The listing builds one solid part. Answer for the finished solid, in the listing's coordinates (mm). Give positions to 0.01 mm unless a question says otherwise; leave off trailing zeros. Write each loop counter-clockwise with the first axis right and the second up, starting at its lowest first coordinate (ties: lowest second). Pieces come first, ordered by that corner, then holes.
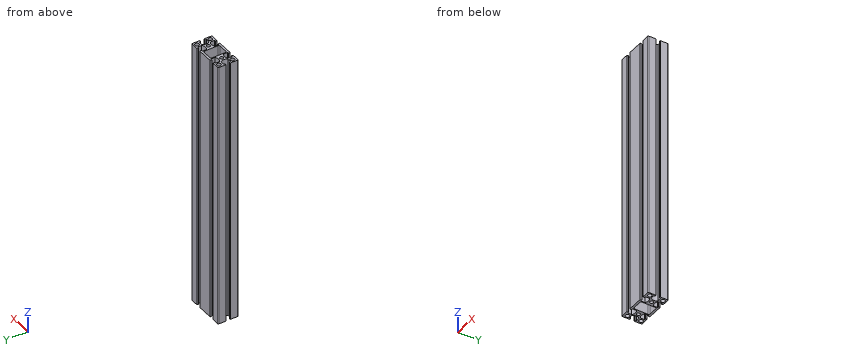
```python
from build123d import *

# Parameters (mm, degrees)
MODEL_R             = 2.5
MODEL_R_2           = 3
BOSS_EXTRUDE1_DEPTH = 400


with BuildPart() as part:
    # Model → Boss-Extrude1 (new body)
    with BuildSketch(Plane.XY):
        with BuildLine():
            Line((-27.5, 3.25), (-30, 3.25))
            Line((-30, 3.25), (-30, 14))
            ThreePointArc((-30, 14), (-29.707106781, 14.707106781), (-29, 15))
            Line((-29, 15), (-18.25, 15))
            Line((-18.25, 15), (-18.25, 12.5))
            Line((-18.25, 12.5), (-20.25, 12.5))
            Line((-20.25, 12.5), (-20.25, 6.643928679))
            ThreePointArc((-20.25, 6.643928679), (-15, 4.5), (-9.75, 6.643928679))
            Line((-9.75, 6.643928679), (-9.75, 12.5))
            Line((-9.75, 12.5), (-11.75, 12.5))
            Line((-11.75, 12.5), (-11.75, 15))
            Line((-11.75, 15), (11.75, 15))
            Line((11.75, 15), (11.75, 12.5))
            Line((11.75, 12.5), (9.75, 12.5))
            Line((9.75, 12.5), (9.75, 6.643928679))
            ThreePointArc((9.75, 6.643928679), (15, 4.5), (20.25, 6.643928679))
            Line((20.25, 6.643928679), (20.25, 12.5))
            Line((20.25, 12.5), (18.25, 12.5))
            Line((18.25, 12.5), (18.25, 15))
            Line((18.25, 15), (29, 15))
            ThreePointArc((29, 15), (29.707106781, 14.707106781), (30, 14))
            Line((30, 14), (30, 3.25))
            Line((30, 3.25), (27.5, 3.25))
            Line((27.5, 3.25), (27.5, 5.25))
            Line((27.5, 5.25), (21.643928679, 5.25))
            ThreePointArc((21.643928679, 5.25), (19.5, 0), (21.643928679, -5.25))
            Line((21.643928679, -5.25), (27.5, -5.25))
            Line((27.5, -5.25), (27.5, -3.25))
            Line((27.5, -3.25), (30, -3.25))
            Line((30, -3.25), (30, -14))
            ThreePointArc((30, -14), (29.707106781, -14.707106781), (29, -15))
            Line((29, -15), (18.25, -15))
            Line((18.25, -15), (18.25, -12.5))
            Line((18.25, -12.5), (20.25, -12.5))
            Line((20.25, -12.5), (20.25, -6.643928679))
            ThreePointArc((20.25, -6.643928679), (15, -4.5), (9.75, -6.643928679))
            Line((9.75, -6.643928679), (9.75, -12.5))
            Line((9.75, -12.5), (11.75, -12.5))
            Line((11.75, -12.5), (11.75, -15))
            Line((11.75, -15), (-11.75, -15))
            Line((-11.75, -15), (-11.75, -12.5))
            Line((-11.75, -12.5), (-9.75, -12.5))
            Line((-9.75, -12.5), (-9.75, -6.643928679))
            ThreePointArc((-9.75, -6.643928679), (-15, -4.5), (-20.25, -6.643928679))
            Line((-20.25, -6.643928679), (-20.25, -12.5))
            Line((-20.25, -12.5), (-18.25, -12.5))
            Line((-18.25, -12.5), (-18.25, -15))
            Line((-18.25, -15), (-29, -15))
            ThreePointArc((-29, -15), (-29.707106781, -14.707106781), (-30, -14))
            Line((-30, -14), (-30, -3.25))
            Line((-30, -3.25), (-27.5, -3.25))
            Line((-27.5, -3.25), (-27.5, -5.25))
            Line((-27.5, -5.25), (-21.643928679, -5.25))
            ThreePointArc((-21.643928679, -5.25), (-19.5, 0), (-21.643928679, 5.25))
            Line((-21.643928679, 5.25), (-27.5, 5.25))
            Line((-27.5, 5.25), (-27.5, 3.25))
        make_face()
        with Locations((-15, 0)):
            Circle(MODEL_R, mode=Mode.SUBTRACT)
        with Locations((-25, 10.531430074)):
            Circle(MODEL_R_2, mode=Mode.SUBTRACT)
        with Locations((-25.399251578, -9.468569926)):
            Circle(MODEL_R_2, mode=Mode.SUBTRACT)
        with Locations((25.399251578, -9.468569926)):
            Circle(MODEL_R_2, mode=Mode.SUBTRACT)
        with Locations((15, 0)):
            Circle(MODEL_R, mode=Mode.SUBTRACT)
        with Locations((25, 10.531430074)):
            Circle(MODEL_R_2, mode=Mode.SUBTRACT)
        with BuildLine():
            Line((6.5, 12), (-6.5, 12))
            ThreePointArc((-6.5, 12), (-7.914213562, 11.414213562), (-8.5, 10))
            Line((-8.5, 10), (-8.5, -10))
            ThreePointArc((-8.5, -10), (-7.914213562, -11.414213562), (-6.5, -12))
            Line((-6.5, -12), (6.5, -12))
            ThreePointArc((6.5, -12), (7.914213562, -11.414213562), (8.5, -10))
            Line((8.5, -10), (8.5, 10))
            ThreePointArc((8.5, 10), (7.914213562, 11.414213562), (6.5, 12))
        make_face(mode=Mode.SUBTRACT)
    extrude(amount=BOSS_EXTRUDE1_DEPTH)


solid = part.part
```
Item 1: Consider probe 1 along X at (y, z) = (-13.25, 230.5); probe 2 along Y at (x, z) = (-25, 177); probe 3 along X at (y, z) = (7, 323). Determine where each line is inside the solid, lowest interval first.
Conclusion:
probe 1: x = -30 to -18.25, -11.75 to 11.75, 18.25 to 30
probe 2: y = -15 to -12.44, -6.5 to -5.25, 5.25 to 7.53, 13.53 to 15
probe 3: x = -30 to -20.25, -9.75 to -8.5, 8.5 to 9.75, 20.25 to 30
Item 2: A cutting plane is placed at B-B, the plane z = 40.5. Count the separate pieces of the cut face and the enclosed holes in it, plus the area to 3 significant figures.
Conclusion:
separate pieces: 1
enclosed holes: 7
area: 683 mm2
Item 3: A cutting plane is placed at A-A, the plane x = 0. Give the vertices of the cut face in (y, z).
Conclusion:
outline: (-15, 0) - (-12, 0) - (-12, 400) - (-15, 400) - close; (12, 0) - (15, 0) - (15, 400) - (12, 400) - close
Item 4: Each of these flat-tipped pins is pushed along its axis until it touches: P1, Ø9.5, axis at x = 25, y = 10.53, coming from the -Z side; P2, Ø3, axis at x = 16.5, z = 130, coming from the -Y side; P3, Ø4, axis at y = -0.5, z = 243, coming from the +X side. Where does it stop, or does it pass through?
Conclusion:
P1: stops at z = 0
P2: stops at y = -5.13
P3: stops at x = 19.93
